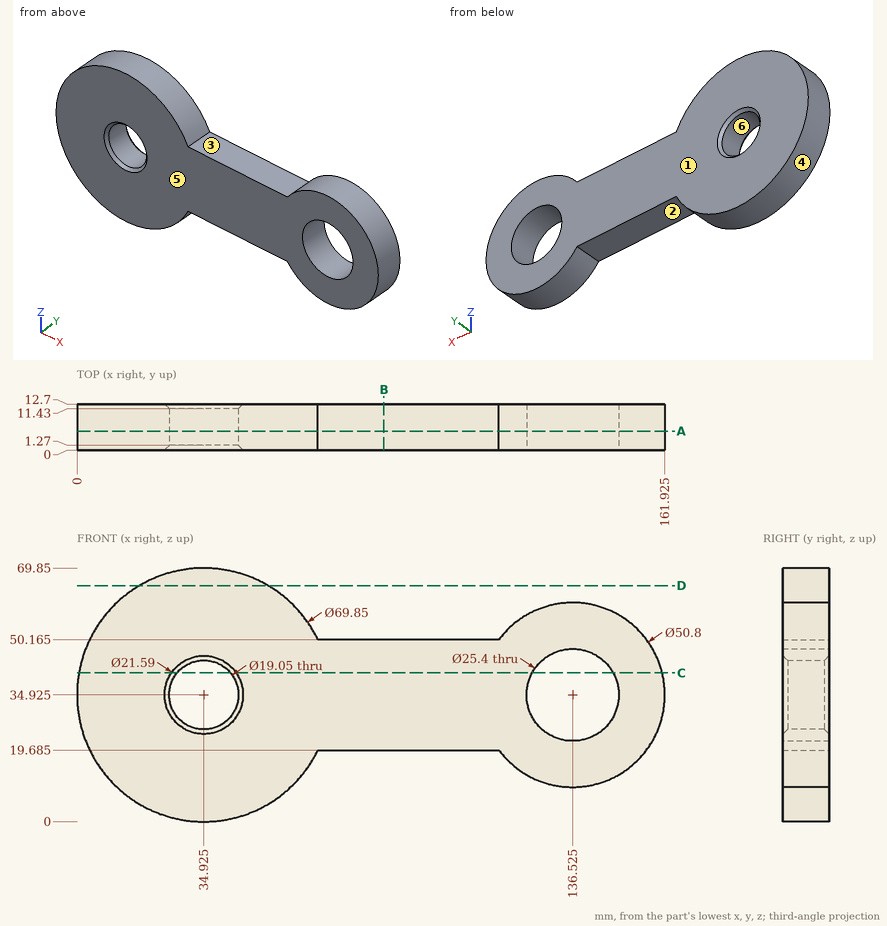
Design review of the part shown in the three views and the two pictorial views. Dimensions are in mm from the part's minimum x, y and z. A direction names the side the tool comes from. Coordinates: 2 decimals unless noted, no trailing zeros. Order: outer loops, then holes, each group sorted by start corner. A loop starts at its lowest first (then second) coordinate and runs counter-clockwise, first axis right, second up. Notation, with made-up numbers: (-30, 13.25) - (-13, 13.25) arc R33 cw to (-13, 51.25) - close; hole circle Ø3 at (-5.75, 50). An arc over 180 degrees is marked (long way). Answer as CSV lines item,"result". Start each with the question number.
1) Machinability: for the marked faces 1, 2 and 3, which of the approach directions +Z, -Z, +X, -X, +Y, -Y give a long, thin tool a straight path to every point of the face, cutting with its end or side? Answer none if there is none.
2) Add section D-D (z = 65). State the section outline as (x, y) points, then the cut area to 3 significant figures.
3) Insertion check: P1, Ø6.5, axis at x = 96, y = 7.5, coming from the -Z side (3 decimals); P2, Ø5, axis at y = 2.5, z = 17.5, coming from the -X side; P3, Ø12, axis at x = 132.5, z = 30, coming from the +Y side; P4, Ø1.5, axis at y = 4, z = 34.5, coming from the -X side. Each pin has a flat end and moves straight along its axis. Give the tip position at first contact, or say it passes through.
4) Add section C-C (z = 41). Count the separate pieces of the cut face and the enclosed holes in it, then the cut area to 3 significant figures.
5) Add section B-B (x = 84.5). State the section outline as (y, z) points (3 decimals).
6) Add section A-A (y = 5.25). State the section outline as (x, z) points (3 decimals).
7) Draft analysis for pull direction Z (two halves, no side actions). For the marked faces 4, 5 and 6, state which applies: +Z half, -Z half, draft (parallel to the pull), parting line (faces both ways), or undercut.
8) To check wall thickness, follow line 1 along Z through (x, y) = (70, 6.5) (3 decimals); line 2 along Z through (x, y) = (132, 10); line 3 along Z through (x, y) = (148, 8.75). State the ranges of each line that lie inside material, in increasing order. Write a range as [from, to].
Result:
1,face 1,"+Z, -Z, +X, -X, +Y"
1,face 2,"-Z, +Y, -Y"
1,face 3,"+Z, +Y, -Y"
2,outline,"(17.17, 0) - (52.68, 0) - (52.68, 12.7) - (17.17, 12.7) - close"
2,area,"451 mm^2"
3,P1,"z = 19.685"
3,P2,"x = 3.35"
3,P3,"through"
3,P4,"x = 0"
4,separate pieces,"3"
4,enclosed holes,"0"
4,area,"1,570 mm^2"
5,outline,"(0, 19.685) - (12.7, 19.685) - (12.7, 50.165) - (0, 50.165) - close"
6,outline,"(66.349, 19.685) - (116.205, 19.685) arc R25.4 ccw (long way) to (116.205, 50.165) - (66.349, 50.165) arc R34.925 ccw (long way) to start; hole circle Ø19.05 at (34.925, 34.925); hole circle Ø25.4 at (136.525, 34.925)"
7,face 4,"parting line"
7,face 5,"draft"
7,face 6,"undercut"
8,line 1,"[19.685, 50.165]"
8,line 2,"[9.93, 23.06], [46.79, 59.92]"
8,line 3,"[12.26, 29.48], [40.37, 57.59]"
